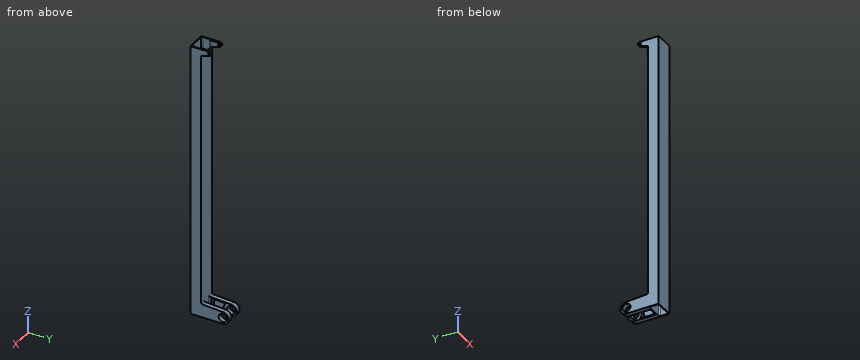
```python
from build123d import *

# Parameters (mm, degrees)
SKETCH2_W               = 177.8
SKETCH2_H               = 101.6
SKETCH2_W_2             = 162.8
SKETCH2_H_2             = 86.6
BOSS_EXTRUDE2_DEPTH     = 2600
SKETCH1_R               = 38.1
BOSS_EXTRUDE3_DEPTH     = 44.45
BOSS_EXTRUDE5_START     = -44.45
SKETCH3_R               = 38.1
BOSS_EXTRUDE5_DEPTH     = 44.45
FILLET1_R               = 12.7
FILLET2_R               = 12.7
SKETCH5_R               = 12.7
BOSS_EXTRUDE7_DEPTH     = 19.05
CUT_EXTRUDE1_DEPTH      = 34.45
CUT_EXTRUDE2_DEPTH      = 2620.044665999
CUT_EXTRUDE2_DEPTH_BACK = 2620.044665999
SKETCH9_W               = 88.9
SKETCH9_H               = 2600
SKETCH10_W              = 137.4
SKETCH10_H              = 75
CUT_EXTRUDE3_DEPTH      = 10


with BuildPart() as part:
    # Sketch2 → Boss-Extrude2 (new body)
    with BuildSketch(Plane.XY):
        with Locations((-88.9, 50.8)):
            Rectangle(SKETCH2_W, SKETCH2_H)
        with Locations((-88.9, 50.8)):
            Rectangle(SKETCH2_W_2, SKETCH2_H_2, mode=Mode.SUBTRACT)
    extrude(amount=BOSS_EXTRUDE2_DEPTH)

    # Sketch1 → Boss-Extrude3 (add)
    with BuildSketch(Plane(origin=(0, 0, 0), x_dir=(0, 0, -1), z_dir=(1, 0, 0))):
        with BuildLine():
            Line((-127, 101.6), (0, 101.6))
            Line((0, 101.6), (0, 304.8))
            ThreePointArc((0, 304.8), (-55.382017361, 361.922646449), (-114.190611982, 308.334272869))
            Line((-114.190611982, 308.334272869), (-127, 101.6))
        make_face()
        with Locations((-57.15, 304.8)):
            Circle(SKETCH1_R, mode=Mode.SUBTRACT)
    extrude(amount=-BOSS_EXTRUDE3_DEPTH)

    # Sketch3 → Boss-Extrude5 (add)
    with BuildSketch(Plane.ZY.offset(177.8).offset(BOSS_EXTRUDE5_START)):
        with BuildLine():
            Line((0, 304.8), (0, 101.6))
            Line((0, 101.6), (127, 101.6))
            Line((127, 101.6), (114.190611982, 308.334272869))
            ThreePointArc((114.190611982, 308.334272869), (55.382017361, 361.922646449), (0, 304.8))
        make_face()
        with Locations(Location((57.15, 304.8, 0), (0, 0, 180))):
            Circle(SKETCH3_R, mode=Mode.SUBTRACT)
    extrude(amount=BOSS_EXTRUDE5_DEPTH)

    # Fillet1
    fillet1_edges = [part.edges().sort_by_distance(p)[0] for p in [
        (-7.5, 94.1, 1300),
        (-170.3, 94.1, 1300),
        (-170.3, 7.5, 1300),
        (-7.5, 7.5, 1300),
    ]]
    fillet(fillet1_edges, radius=FILLET1_R)

    # Fillet2
    fillet2_edges = [part.edges().sort_by_distance(p)[0] for p in [
        (-44.45, 101.6, 63.5),
        (-22.225, 101.6, 127),
        (-133.35, 101.6, 63.5),
        (-155.575, 101.6, 127),
    ]]
    fillet(fillet2_edges, radius=FILLET2_R)

    # Sketch5 → Boss-Extrude7 (add)
    with BuildSketch(Plane(origin=(0, 0, 0), x_dir=(0, 0, -1), z_dir=(1, 0, 0))):
        with BuildLine():
            Line((-2600, 101.6), (-2600, 180.34))
            ThreePointArc((-2600, 180.34), (-2583.812295525, 199.173740052), (-2562.760129729, 185.999604185))
            Line((-2562.760129729, 185.999604185), (-2536.5, 101.6))
            Line((-2536.5, 101.6), (-2600, 101.6))
        make_face()
        with Locations((-2580.95, 180.34)):
            Circle(SKETCH5_R, mode=Mode.SUBTRACT)
    boss_extrude7 = extrude(amount=-BOSS_EXTRUDE7_DEPTH)

    # Mirror1: Boss-Extrude7 across plane
    add(boss_extrude7.mirror(Plane.ZY.offset(88.9)))

    # Sketch8 → Cut-Extrude1 (cut)
    with BuildSketch(Plane(origin=(-133.35, 0, 0), x_dir=(0, 0, -1), z_dir=(1, 0, 0))):
        with BuildLine():
            ThreePointArc((-10, 255.662565187), (-59.256729969, 236.73259452), (-107.248511945, 258.672469165))
            Line((-107.248511945, 258.672469165), (-115.574316238, 124.3))
            Line((-115.574316238, 124.3), (-10, 124.3))
            Line((-10, 124.3), (-10, 255.662565187))
        make_face()
    extrude(amount=-CUT_EXTRUDE1_DEPTH, mode=Mode.SUBTRACT)

    # Sketch9 → Cut-Extrude2 (cut, two sides: drawn at the far end of the back side and taken through both)
    with BuildSketch(Plane(origin=(0, 101.6, 0), x_dir=(1, 0, 0), z_dir=(0, 1, 0)).offset(-CUT_EXTRUDE2_DEPTH_BACK)):
        with Locations((-44.45, -1300)):
            Rectangle(SKETCH9_W, SKETCH9_H)
    extrude(amount=CUT_EXTRUDE2_DEPTH + CUT_EXTRUDE2_DEPTH_BACK, mode=Mode.SUBTRACT)

    # Mirror2: part across plane


with BuildPart() as part_1:
    add(part.part)
    add(part.part.mirror(Plane.ZY.offset(88.9)))

    # Sketch10 → Cut-Extrude3 (cut)
    with BuildSketch(Plane.XZ.offset(-94.1)):
        with Locations((-88.9, 2562.5)):
            Rectangle(SKETCH10_W, SKETCH10_H)
    extrude(amount=-CUT_EXTRUDE3_DEPTH, mode=Mode.SUBTRACT)


solid = part_1.part
```
Design review of the part built by this model. Coordinates are the model's own, in mm. Give positions to 0.01 mm unless a question says otherwise; leave off trailing zeros. Return JSON: item names as keys, results as strings. Group by question number.
(1) To check wall thickness, follow probe 1 along Y at (x, z) = (-29, 57.15); probe 2 along Z at (x, y) = (-165, 304); probe 3 along Y at (x, z) = (-151, 1376.5). State the ranges of each line that lie inside material, in increasing order.
(2) We need section A-A, the plane z = 57.15. Give the number of separate pieces and of enclosed holes in the cut face, then the cut area to 3 significant figures.
(3) Insertion check: pin 1 (2 mm diameter, centred on x = -106.5, z = 401.5, fed in from +Y); pin 2 (17 mm diameter, centred on x = -34.5, z = 88.5, fed in from +Y). Each pin has a flat end and moves straight along its axis. Give the tip position at first contact, or say it passes through.
Reported:
{
 "1": {"probe 1": "y = 0 to 7.5, 94.1 to 124.3, 236.7 to 266.7, 342.9 to 361.95", "probe 2": "z = 0 to 19.06, 95.24 to 114.46", "probe 3": "y = 0 to 7.5, 94.1 to 101.6"},
 "2": {"separate pieces": "3", "enclosed holes": "1", "area": "12,800 mm2"},
 "3": {"pin 1": "stops at y = 101.6", "pin 2": "stops at y = 357.18"}
}
